from build123d import *

# Parameters (mm, degrees)
SKETCH1_R           = 3.96875
SKETCH1_R_2         = 1.984375
BOSS_EXTRUDE1_DEPTH = 3.175
FILLET1_R           = 0.1
SKETCH2_R           = 3.86875
SKETCH2_R_2         = 2.084375
CUT_EXTRUDE1_DEPTH  = 0.5
SKETCH3_R           = 3.86875
SKETCH3_R_2         = 2.084375
CUT_EXTRUDE2_DEPTH  = 0.5


with BuildPart() as part:
    # Sketch1 → Boss-Extrude1 (new body)
    with BuildSketch(Plane(origin=(0, 0, 0), x_dir=(1, 0, 0), z_dir=(0, 1, 0))):
        Circle(SKETCH1_R)
        Circle(SKETCH1_R_2, mode=Mode.SUBTRACT)
    extrude(amount=BOSS_EXTRUDE1_DEPTH)

    # Fillet1
    fillet1_edges = [part.edges().sort_by_distance(p)[0] for p in [
        (-3.96875, 0, 0),
        (-3.96875, 3.175, 0),
        (-1.984375, 0, 0),
        (-1.984375, 3.175, 0),
    ]]
    fillet(fillet1_edges, radius=FILLET1_R)

    # Sketch2 → Cut-Extrude1 (cut)
    with BuildSketch(Plane(origin=(0, 3.175, 0), x_dir=(1, 0, 0), z_dir=(0, 1, 0))):
        Circle(SKETCH2_R)
        Circle(SKETCH2_R_2, mode=Mode.SUBTRACT)
    extrude(amount=-CUT_EXTRUDE1_DEPTH, mode=Mode.SUBTRACT)

    # Sketch3 → Cut-Extrude2 (cut)
    with BuildSketch(Plane.XZ):
        Circle(SKETCH3_R)
        Circle(SKETCH3_R_2, mode=Mode.SUBTRACT)
    extrude(amount=-CUT_EXTRUDE2_DEPTH, mode=Mode.SUBTRACT)


solid = part.part
Work out the finished part from the listing and answer in its coordinate system (mm). Coordinates: 2 decimals unless noted, no trailing zeros. Loops run counter-clockwise (first coordinate to the right, second up) from the corner with the lowest first, then second, coordinate; pieces in that order, holes last. Notation, with made-up numbers: (-39, -0.5) -> (19, -0.5) arc R17 cw to (19, 4.5) -> close; hole circle Ø9 at (48.25, 3). An arc over 180 degrees is marked (long way). Write each question's results on one line, items separated by ' | '. Start each with the question number.
1) Consider line 1 along Z through (x, y) = (0, 2.35); line 2 along X through (y, z) = (3.05, -3.5). Determine where each line is inside the solid, lowest interval first.
2) Find section A-A on x = 0. Determine the outline of the cut face in (y, z) (3 decimals), then the cut area to 3 significant figures.
3) The mould has two halves that part along Z. Classify faces 1 (the cylindrical face through (-0.43, 1.567, 1.937)), 2 (the cylindrical face through (-0.86, 1.567, 3.874)), 3 (the flat face through (2, 0.5, -2)): pulls with the +Z half, pulls with the -Z half, needs draft (parallel to the pull), parting line crosses it, or undercut.
4) Flat-ended cylindrical pins translate along their axes: P1, Ø2, axis at x = 0.5, z = -2.5, coming from the +Y side (3 decimals); P2, Ø1.5, axis at y = 2, z = -3, coming from the +X side. Find the tip coordinate at first contact, or state that the pin passes through.
5) Find section B-B on z = 0. Determine the outline of the cut face in (x, y) (3 decimals).
6) Find section C-C on y = 2.1. Determine the outline of the cut face in (x, z).
Response values:
1) line 1: z = -3.97 to -1.98, 1.98 to 3.97 | line 2: x = -1.87 to -1.65, 1.65 to 1.87
2) outline: (0, -3.869) arc R0.1 ccw to (0.1, -3.969) -> (3.075, -3.969) arc R0.1 ccw to (3.175, -3.869) -> (2.675, -3.869) -> (2.675, -2.084) -> (3.175, -2.084) arc R0.1 ccw to (3.075, -1.984) -> (0.1, -1.984) arc R0.1 ccw to (0, -2.084) -> (0.5, -2.084) -> (0.5, -3.869) -> close; (0, 2.084) arc R0.1 ccw to (0.1, 1.984) -> (3.075, 1.984) arc R0.1 ccw to (3.175, 2.084) -> (2.675, 2.084) -> (2.675, 3.869) -> (3.175, 3.869) arc R0.1 ccw to (3.075, 3.969) -> (0.1, 3.969) arc R0.1 ccw to (0, 3.869) -> (0.5, 3.869) -> (0.5, 2.084) -> close | area: 9.01 mm^2
3) face 1: undercut | face 2: parting line crosses it | face 3: undercut
4) P1: stops at y = 3.175 | P2: stops at x = 3.27
5) outline: (-3.969, 0.1) arc R0.1 ccw to (-3.869, 0) -> (-3.869, 0.5) -> (-2.084, 0.5) -> (-2.084, 0) arc R0.1 ccw to (-1.984, 0.1) -> (-1.984, 3.075) arc R0.1 ccw to (-2.084, 3.175) -> (-2.084, 2.675) -> (-3.869, 2.675) -> (-3.869, 3.175) arc R0.1 ccw to (-3.969, 3.075) -> close; (1.984, 0.1) arc R0.1 ccw to (2.084, 0) -> (2.084, 0.5) -> (3.869, 0.5) -> (3.869, 0) arc R0.1 ccw to (3.969, 0.1) -> (3.969, 3.075) arc R0.1 ccw to (3.869, 3.175) -> (3.869, 2.675) -> (2.084, 2.675) -> (2.084, 3.175) arc R0.1 ccw to (1.984, 3.075) -> close
6) outline: circle Ø7.94 at (0, 0); hole circle Ø3.97 at (0, 0)
